Could you check a few things on this model? Use its own coordinates, in mm. Face numbers are marked on the shaded views. A direction names the side the tool comes from. Coordinates: 2 decimals unless noted, no trailing zeros. Loops run counter-clockwise (first coordinate to the right, second up) from the corner with the lowest first, then second, coordinate; pieces in that order, holes last. Notation, with made-up numbers: (49, 73.25) -> (71, 73.25) arc R21 cw to (71, 110.25) -> close; hole circle Ø1 at (11.5, -31.5). An arc over 180 degrees is marked (long way). One line per question, with ' | ' between items. Start each with the question number.
(1) Which directions (+Z, -Z, +X, -X, +Y, -Y) give clear straight access to the entire face, cutting with the end or side of a thin tool? Please do the marked faces 4, 5, 6, 7 and 8.
(2) If we mould it in two halves opening along Y, with no side actions, what happens to the marked faces 1, 2 and 3? For each: pulls with the +Y half, pulls with the -Y half, needs draft (parallel to the pull), parting line crosses it, or undercut.
(3) Suppose I cut it at C-C (z = 21). Give the number of separate pieces and of enclosed holes in the cut face, plus the area to 3 significant figures.
(4) Suppose I cut it at B-B (x = -15.5). Please give me the cut outline in (y, z).
(5) If I drill on line 1 along X through (y, z) = (-6.5, 7.5); line 2 along Y through (x, z) = (-5, 2); line 3 along X through (y, z) = (-16, 21.5), over which ranges is the centre line in solid material (lowest first)?
(6) I'm going to push flat-ended pins straight in: pin 1 Ø10 at (y, z) = (0, 11.5) entering from +X; pin 2 Ø8 at (x, y) = (-42.5, 11) entering from +Z; pin 3 Ø3 at (x, y) = (-30, 30) entering from -Z. Where does each tip first touch, or does it pass through?
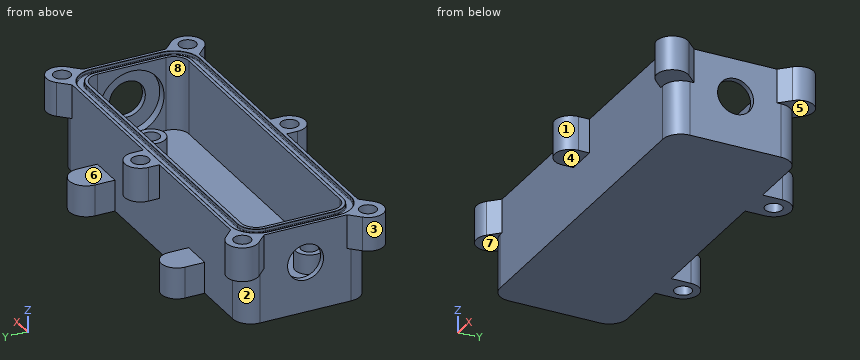
```python
from build123d import *

# Parameters (mm, degrees)
SKETCH1_W               = 114.3
SKETCH1_H               = 34.925
BOSS_EXTRUDE1_DEPTH     = 26
SHELL1_T                = 5
FILLET1_R               = 5.334
FILLET2_R               = 6.35
CUT_EXTRUDE1_DEPTH      = 1.2446
FILLET3_R               = 0.254
FILLET4_R               = 0.127
BOSS_EXTRUDE3_START     = -12
BOSS_EXTRUDE3_DEPTH     = 12
SKETCH5_R               = 3.025
CUT_EXTRUDE3_DEPTH      = 9
MIRROR2_START           = -12
MIRROR2_COPY_1_DEPTH    = 12
MIRROR2_COPY_2_SKETCH_R = 3.025
MIRROR2_COPY_2_DEPTH    = 9
BOSS_EXTRUDE4_DEPTH     = 12
SKETCH7_R               = 3.025
CUT_EXTRUDE4_DEPTH      = 9
CUT_EXTRUDE5_DEPTH      = 6
SKETCH10_R              = 5
SKETCH10_R_2            = 3.025
BOSS_EXTRUDE5_DEPTH     = 7
SKETCH11_R              = 11.43
CUT_EXTRUDE6_DEPTH      = 3
SKETCH12_R              = 6
SKETCH12_R_2            = 3.025
SKETCH12_R_3            = 5.5
BOSS_EXTRUDE6_DEPTH     = 11
SKETCH13_R              = 3.025
CUT_EXTRUDE7_DEPTH      = 9


with BuildPart() as part:
    # Sketch1 → Boss-Extrude1 (new body)
    with BuildSketch(Plane.XY):
        Rectangle(SKETCH1_W, SKETCH1_H)
    extrude(amount=BOSS_EXTRUDE1_DEPTH)

    # Shell1
    shell1_openings = [part.faces().sort_by_distance(p)[0] for p in [
        (0, 0, 26),
    ]]
    offset(amount=SHELL1_T, openings=shell1_openings, kind=Kind.INTERSECTION)

    # Fillet1
    # the kernel refuses this fillet: 5.334 mm, written as the material it adds along each edge
    with BuildSketch(Plane(origin=(57.15, -17.4625, 0), x_dir=(0, 1, 0), z_dir=(0, 0, 1)), Plane(origin=(57.15, 17.4625, 0), x_dir=(-1, 0, 0), z_dir=(0, 0, 1)), Plane(origin=(-57.15, -17.4625, 0), x_dir=(1, 0, 0), z_dir=(0, 0, 1))) as fillet1_piece_1:
        with BuildLine():
            CenterArc((FILLET1_R, FILLET1_R), FILLET1_R, 180, 90)
            Line((0, FILLET1_R), (0, 0))
            Line((0, 0), (FILLET1_R, 0))
        make_face()
    extrude(amount=26)
    with BuildSketch(Plane(origin=(-57.15, 17.4625, 0), x_dir=(1, 0, 0), z_dir=(0, 0, 1))) as fillet1_piece_2:
        with BuildLine():
            CenterArc((FILLET1_R, -FILLET1_R), FILLET1_R, 90, 90)
            Line((0, -FILLET1_R), (0, 0))
            Line((0, 0), (FILLET1_R, 0))
        make_face()
    extrude(amount=26)

    # Fillet2
    fillet2_edges = [part.edges().sort_by_distance(p)[0] for p in [
        (62.15, -22.4625, 10.5),
        (-62.15, -22.4625, 10.5),
        (-62.15, 22.4625, 10.5),
        (62.15, 22.4625, 10.5),
    ]]
    fillet(fillet2_edges, radius=FILLET2_R)

    # Sketch2 → Cut-Extrude1 (cut)
    with BuildSketch(Plane.XY.offset(26)):
        with BuildLine():
            Line((-60.9327, 12.1285), (-60.9327, -12.1285))
            ThreePointArc((-60.9327, -12.1285), (-58.262480392, -18.574980392), (-51.816, -21.2452))
            Line((-51.816, -21.2452), (51.816, -21.2452))
            ThreePointArc((51.816, -21.2452), (58.262480392, -18.574980392), (60.9327, -12.1285))
            Line((60.9327, -12.1285), (60.9327, 12.1285))
            ThreePointArc((60.9327, 12.1285), (58.262480392, 18.574980392), (51.816, 21.2452))
            Line((51.816, 21.2452), (-51.816, 21.2452))
            ThreePointArc((-51.816, 21.2452), (-58.262480392, 18.574980392), (-60.9327, 12.1285))
        make_face()
        with BuildLine():
            Line((51.816, 18.6798), (-51.816, 18.6798))
            ThreePointArc((-51.816, 18.6798), (-56.448468656, 16.760968656), (-58.3673, 12.1285))
            Line((-58.3673, 12.1285), (-58.3673, -12.1285))
            ThreePointArc((-58.3673, -12.1285), (-56.448468656, -16.760968656), (-51.816, -18.6798))
            Line((-51.816, -18.6798), (51.816, -18.6798))
            ThreePointArc((51.816, -18.6798), (56.448468656, -16.760968656), (58.3673, -12.1285))
            Line((58.3673, -12.1285), (58.3673, 12.1285))
            ThreePointArc((58.3673, 12.1285), (56.448468656, 16.760968656), (51.816, 18.6798))
        make_face(mode=Mode.SUBTRACT)
    extrude(amount=-CUT_EXTRUDE1_DEPTH, mode=Mode.SUBTRACT)

    # Fillet3
    fillet3_edges = [part.edges().sort_by_distance(p)[0] for p in [
        (-58.262480392, 18.574980392, 24.7554),
        (0, 21.2452, 24.7554),
        (58.262480392, 18.574980392, 24.7554),
        (60.9327, 0, 24.7554),
        (58.262480392, -18.574980392, 24.7554),
        (0, -21.2452, 24.7554),
        (-58.262480392, -18.574980392, 24.7554),
        (-60.9327, 0, 24.7554),
        (58.3673, 0, 24.7554),
        (56.448468656, 16.760968656, 24.7554),
        (0, 18.6798, 24.7554),
        (-56.448468656, 16.760968656, 24.7554),
        (-58.3673, 0, 24.7554),
        (-56.448468656, -16.760968656, 24.7554),
        (0, -18.6798, 24.7554),
        (56.448468656, -16.760968656, 24.7554),
    ]]
    fillet(fillet3_edges, radius=FILLET3_R)

    # Fillet4
    fillet4_edges = [part.edges().sort_by_distance(p)[0] for p in [
        (-58.262480392, 18.574980392, 26),
        (-60.9327, 0, 26),
        (-58.262480392, -18.574980392, 26),
        (0, -21.2452, 26),
        (58.262480392, -18.574980392, 26),
        (60.9327, 0, 26),
        (58.262480392, 18.574980392, 26),
        (0, 21.2452, 26),
        (56.448468656, 16.760968656, 26),
        (58.3673, 0, 26),
        (56.448468656, -16.760968656, 26),
        (0, -18.6798, 26),
        (-56.448468656, -16.760968656, 26),
        (-58.3673, 0, 26),
        (-56.448468656, 16.760968656, 26),
        (0, 18.6798, 26),
    ]]
    fillet(fillet4_edges, radius=FILLET4_R)

    # Sketch4 → Boss-Extrude3 (add)
    with BuildSketch(Plane.XY.offset(26).offset(BOSS_EXTRUDE3_START)):
        with BuildLine():
            ThreePointArc((62.15, -16.1125), (61.666635031, -18.542539796), (60.290128061, -20.602628061))
            ThreePointArc((60.290128061, -20.602628061), (58.230039796, -21.979135031), (55.8, -22.4625))
            Line((55.8, -22.4625), (54.371825407, -22.4625))
            Line((54.371825407, -22.4625), (57.998729563, -26.089404156))
            ThreePointArc((57.998729563, -26.089404156), (65.776904156, -26.089404156), (65.776904156, -18.311229563))
            Line((65.776904156, -18.311229563), (62.15, -14.684325407))
            Line((62.15, -14.684325407), (62.15, -16.1125))
        make_face()
    boss_extrude3 = extrude(amount=BOSS_EXTRUDE3_DEPTH)

    # Sketch5 → Cut-Extrude3 (cut)
    with BuildSketch(Plane.XY.offset(26)):
        with Locations((61.887816859, -22.200316859)):
            Circle(SKETCH5_R)
    cut_extrude3 = extrude(amount=-CUT_EXTRUDE3_DEPTH, mode=Mode.SUBTRACT)

    # Mirror1: Boss-Extrude3, Cut-Extrude3 across plane
    add(boss_extrude3.mirror(Plane.ZX))
    add(cut_extrude3.mirror(Plane.ZX), mode=Mode.SUBTRACT)

    # Mirror2: Boss-Extrude3, Cut-Extrude3 across plane
    add(boss_extrude3.mirror(Plane(origin=(0, 0, 0), x_dir=(0, 0, 1), z_dir=(1, 0, 0))))
    add(cut_extrude3.mirror(Plane(origin=(0, 0, 0), x_dir=(0, 0, 1), z_dir=(1, 0, 0))), mode=Mode.SUBTRACT)

    # Mirror2 copy 1 sketch → Mirror2 copy 1 (add)
    with BuildSketch(Plane(origin=(0, 0, 26), x_dir=(-1, 0, 0), z_dir=(0, 0, 1)).offset(MIRROR2_START)):
        with BuildLine():
            ThreePointArc((62.15, -16.1125), (61.666635031, -18.542539796), (60.290128061, -20.602628061))
            ThreePointArc((60.290128061, -20.602628061), (58.230039796, -21.979135031), (55.8, -22.4625))
            Line((55.8, -22.4625), (54.371825407, -22.4625))
            Line((54.371825407, -22.4625), (57.998729563, -26.089404156))
            ThreePointArc((57.998729563, -26.089404156), (65.776904156, -26.089404156), (65.776904156, -18.311229563))
            Line((65.776904156, -18.311229563), (62.15, -14.684325407))
            Line((62.15, -14.684325407), (62.15, -16.1125))
        make_face()
    extrude(amount=MIRROR2_COPY_1_DEPTH)

    # Mirror2 copy 2 sketch → Mirror2 copy 2 (cut)
    with BuildSketch(Plane(origin=(0, 0, 26), x_dir=(-1, 0, 0), z_dir=(0, 0, 1))):
        with Locations((61.887816859, -22.200316859)):
            Circle(MIRROR2_COPY_2_SKETCH_R)
    extrude(amount=-MIRROR2_COPY_2_DEPTH, mode=Mode.SUBTRACT)

    # Sketch6 → Boss-Extrude4 (add)
    with BuildSketch(Plane.XY.offset(26)):
        with BuildLine():
            Line((0, -22.4625), (-5.5, -22.4625))
            Line((-5.5, -22.4625), (-5.5, -26.3722))
            ThreePointArc((-5.5, -26.3722), (0, -31.8722), (5.5, -26.3722))
            Line((5.5, -26.3722), (5.5, -22.4625))
            Line((5.5, -22.4625), (0, -22.4625))
        make_face()
    boss_extrude4 = extrude(amount=-BOSS_EXTRUDE4_DEPTH)

    # Sketch7 → Cut-Extrude4 (cut)
    with BuildSketch(Plane.XY.offset(26)):
        with Locations((0, -26.3722)):
            Circle(SKETCH7_R)
    cut_extrude4 = extrude(amount=-CUT_EXTRUDE4_DEPTH, mode=Mode.SUBTRACT)

    # Mirror3: Boss-Extrude4, Cut-Extrude4 across plane
    add(boss_extrude4.mirror(Plane.ZX))
    add(cut_extrude4.mirror(Plane.ZX), mode=Mode.SUBTRACT)

    # Sketch9 → Cut-Extrude5 (cut)
    with BuildSketch(Plane(origin=(62.15, 0, 0), x_dir=(0, 0, -1), z_dir=(1, 0, 0))):
        with BuildLine():
            ThreePointArc((-19.05, 0), (-12.7, -6.35), (-6.35, 0))
            Line((-6.35, 0), (-19.05, 0))
        make_face()
        with BuildLine():
            Line((-19.05, 0), (-6.35, 0))
            ThreePointArc((-6.35, 0), (-12.7, 6.35), (-19.05, 0))
        make_face()
    cut_extrude5 = extrude(amount=-CUT_EXTRUDE5_DEPTH, mode=Mode.SUBTRACT)

    # Sketch10 → Boss-Extrude5 (add)
    # profile 1 of 3: a face of its own
    with BuildSketch(Plane.XY):
        with Locations((-44.513500214, 10.477500595)):
            Circle(SKETCH10_R)
        with Locations((-44.513500214, 10.477500595)):
            Circle(SKETCH10_R_2, mode=Mode.SUBTRACT)
    # profile 2 of 3: a face of its own
    with BuildSketch(Plane.XY):
        with Locations((-44.513500214, -10.477499405)):
            Circle(SKETCH10_R)
        with Locations((-44.513500214, -10.477499405)):
            Circle(SKETCH10_R_2, mode=Mode.SUBTRACT)
    # profile 3 of 3: a face of its own
    with BuildSketch(Plane.XY):
        with Locations((44.126499786, -0.097499405)):
            Circle(SKETCH10_R)
        with Locations((44.126499786, -0.097499405)):
            Circle(SKETCH10_R_2, mode=Mode.SUBTRACT)
    extrude(amount=BOSS_EXTRUDE5_DEPTH)

    # Sketch11 → Cut-Extrude6 (cut)
    with BuildSketch(Plane.ZY.offset(-57.15)):
        with Locations((12.7, 0)):
            Circle(SKETCH11_R)
    cut_extrude6 = extrude(amount=-CUT_EXTRUDE6_DEPTH, mode=Mode.SUBTRACT)

    # Mirror4: Cut-Extrude5, Cut-Extrude6 across plane
    add(cut_extrude5.mirror(Plane(origin=(0, 0, 0), x_dir=(0, 0, 1), z_dir=(1, 0, 0))), mode=Mode.SUBTRACT)
    add(cut_extrude6.mirror(Plane(origin=(0, 0, 0), x_dir=(0, 0, 1), z_dir=(1, 0, 0))), mode=Mode.SUBTRACT)

    # Sketch12 → Boss-Extrude6 (add)
    # profile 1 of 6: a face of its own
    with BuildSketch(Plane(origin=(0, 0, -5), x_dir=(-1, 0, 0), z_dir=(0, 0, -1))):
        with BuildLine():
            Line((-37.075, 29.4625), (-37.075, 22.4625))
            Line((-37.075, 22.4625), (-31.075, 22.4625))
            Line((-31.075, 22.4625), (-25.075, 22.4625))
            Line((-25.075, 22.4625), (-25.075, 29.4625))
            ThreePointArc((-25.075, 29.4625), (-31.075, 23.4625), (-37.075, 29.4625))
        make_face()
    # profile 2 of 6: a face of its own
    with BuildSketch(Plane(origin=(0, 0, -5), x_dir=(-1, 0, 0), z_dir=(0, 0, -1))):
        with Locations((-31.075, 29.4625)):
            Circle(SKETCH12_R)
        with Locations((-31.075, 29.4625)):
            Circle(SKETCH12_R_2, mode=Mode.SUBTRACT)
    # profile 3 of 6: a face of its own
    with BuildSketch(Plane(origin=(0, 0, -5), x_dir=(-1, 0, 0), z_dir=(0, 0, -1))):
        with Locations((-31.075, 29.4625)):
            Circle(SKETCH12_R_2)
    # profile 4 of 6: a face of its own
    with BuildSketch(Plane(origin=(0, 0, -5), x_dir=(-1, 0, 0), z_dir=(0, 0, -1))):
        with BuildLine():
            Line((25.575, 29.4625), (25.575, 22.4625))
            Line((25.575, 22.4625), (36.575, 22.4625))
            Line((36.575, 22.4625), (36.575, 29.4625))
            ThreePointArc((36.575, 29.4625), (31.075, 23.9625), (25.575, 29.4625))
        make_face()
    # profile 5 of 6: a face of its own
    with BuildSketch(Plane(origin=(0, 0, -5), x_dir=(-1, 0, 0), z_dir=(0, 0, -1))):
        with Locations((31.075, 29.4625)):
            Circle(SKETCH12_R_3)
        with Locations((31.075, 29.4625)):
            Circle(SKETCH12_R_2, mode=Mode.SUBTRACT)
    # profile 6 of 6: a face of its own
    with BuildSketch(Plane(origin=(0, 0, -5), x_dir=(-1, 0, 0), z_dir=(0, 0, -1))):
        with Locations((31.075, 29.4625)):
            Circle(SKETCH12_R_2)
    extrude(amount=-BOSS_EXTRUDE6_DEPTH)

    # Sketch13 → Cut-Extrude7 (cut)
    with BuildSketch(Plane(origin=(0, 0, -5), x_dir=(-1, 0, 0), z_dir=(0, 0, -1))):
        with Locations((-31.075, 29.4625)):
            Circle(SKETCH13_R)
        with Locations((31.075, 29.4625)):
            Circle(SKETCH13_R)
    extrude(amount=-CUT_EXTRUDE7_DEPTH, mode=Mode.SUBTRACT)


solid = part.part
```
Checks:
1) face 4: -Z, +X, -X, -Y | face 5: -Z, +X, +Y | face 6: +Z, +X, -X, +Y | face 7: -Z, -X, -Y | face 8: +Z
2) face 1: pulls with the -Y half | face 2: pulls with the +Y half | face 3: undercut
3) separate pieces: 1 | enclosed holes: 7 | area: 1,830 mm^2
4) outline: (-22.46, -5) -> (22.46, -5) -> (22.46, 26) -> (21.37, 26) arc R0.13 ccw to (21.25, 25.87) -> (21.25, 25.01) arc R0.25 cw to (20.99, 24.76) -> (18.93, 24.76) arc R0.25 cw to (18.68, 25.01) -> (18.68, 25.87) arc R0.13 ccw to (18.55, 26) -> (17.46, 26) -> (17.46, 0) -> (-17.46, 0) -> (-17.46, 26) -> (-18.55, 26) arc R0.13 ccw to (-18.68, 25.87) -> (-18.68, 25.01) arc R0.25 cw to (-18.93, 24.76) -> (-20.99, 24.76) arc R0.25 cw to (-21.25, 25.01) -> (-21.25, 25.87) arc R0.13 ccw to (-21.37, 26) -> (-22.46, 26) -> close
5) line 1: x = -62.15 to -60.15, 60.15 to 62.15 | line 2: y = -22.46 to -17.46, 17.46 to 22.46 | line 3: x = -63.47 to -55.49, 55.49 to 63.47
6) pin 1: stops at x = 49.13 | pin 2: stops at z = 7 | pin 3: stops at z = 4
